Geometry: see drawing. Coordinates: mm, zero at the bounding-box minimum. Give positions to 0.01 mm unless a question says otherwise; leave off trailing zeros. Write each loop counter-clockwise with the first axis right and the second up, starting at its lowest first coordinate (ties: lowest second). Pieces come first, ordered by that corner, then holes. Notation, with made-up numbers: (-29.5, 5) - (2.5, 5) arc R29 ccw to (2.5, 26) - close; hole circle Ø8 at (-39.75, 81.25). An arc over 180 degrees is marked (long way). Return JSON: item names as keys, results as strings.
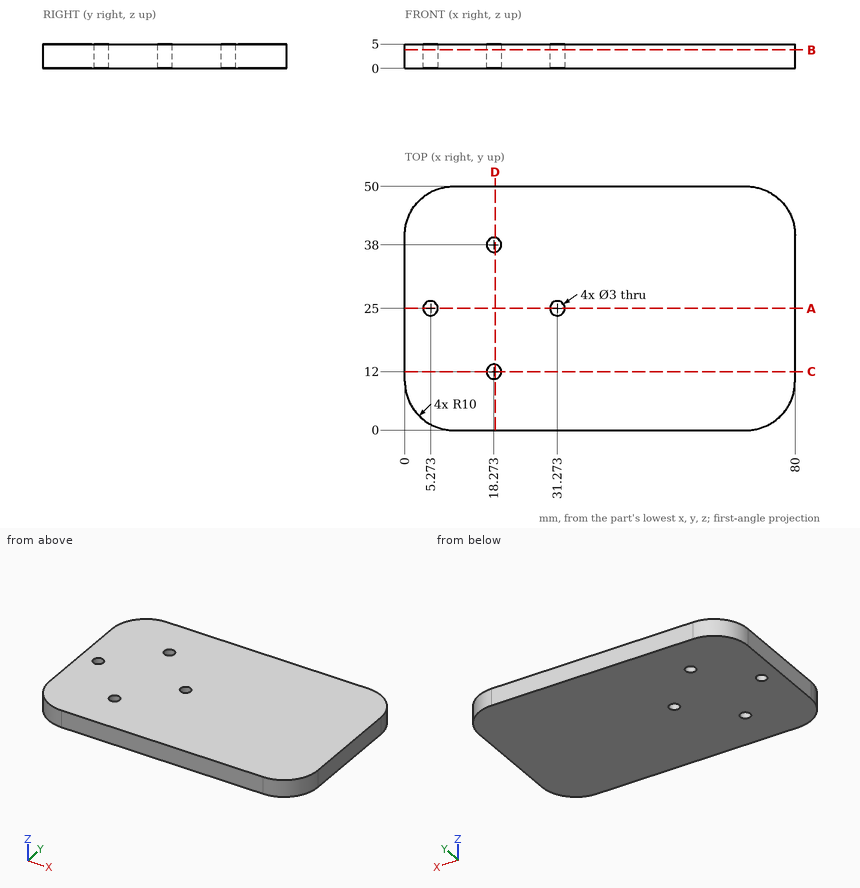
Q1. Section query B-B, the plane z = 3.8. Return the cut outline in (x, y), plus the area to 3 significant figures.
Answer key:
{"outline": "(0, 10) arc R10 ccw to (10, 0) - (70, 0) arc R10 ccw to (80, 10) - (80, 40) arc R10 ccw to (70, 50) - (10, 50) arc R10 ccw to (0, 40) - close; hole circle Ø3 at (5.27, 25); hole circle Ø3 at (18.27, 12); hole circle Ø3 at (18.27, 38); hole circle Ø3 at (31.27, 25)", "area": "3,890 mm^2"}
Q2. Material intervals for probe 1 along Y at (x, z) = (4.5, 4.35) (1 decimal); probe 2 along X at (y, z) = (38.5, 3.85); probe 3 along Y at (x, z) = (9.5, 4.3), sorted ascending. Write a range as [from, to].
Answer key:
{"probe 1": "y = [1.6, 23.7], [26.3, 48.4]", "probe 2": "x = [0, 16.86], [19.69, 80]", "probe 3": "y = [0.01, 49.99]"}
Q3. Section query C-C, the plane y = 12. Return the cut outline in (x, z).
Answer key:
{"outline": "(0, 0) - (16.77, 0) - (16.77, 5) - (0, 5) - close; (19.77, 0) - (80, 0) - (80, 5) - (19.77, 5) - close"}
Q4. Section query D-D, the plane x = 18.5. Return the cut outline in (y, z), plus the area to 3 significant figures.
Answer key:
{"outline": "(0, 0) - (10.52, 0) - (10.52, 5) - (0, 5) - close; (13.48, 0) - (36.52, 0) - (36.52, 5) - (13.48, 5) - close; (39.48, 0) - (50, 0) - (50, 5) - (39.48, 5) - close", "area": "220 mm^2"}
Q5. Section query A-A, the plane y = 25. Return the cut outline in (x, z).
Answer key:
{"outline": "(0, 0) - (3.77, 0) - (3.77, 5) - (0, 5) - close; (6.77, 0) - (29.77, 0) - (29.77, 5) - (6.77, 5) - close; (32.77, 0) - (80, 0) - (80, 5) - (32.77, 5) - close"}
